from build123d import *

# Parameters (mm, degrees)
SKETCH_1_R                      = 4
EXTRUDE_1_DEPTH                 = 1
SKETCH_3_R                      = 2
EXTRUDE_3_DEPTH                 = 6.4
EXTRUDE_4_DEPTH                 = 2
CHAMFER_1_SIZE                  = 0.5
CHAMFER_2_SIZE                  = 1
CUT_EXTRUDE_1_REACH             = 10.542
CUT_EXTRUDE_1_DIRECTION_2_REACH = 10.542
EXTRUDE_START                   = 0.6
SKETCH_6_R                      = 4
EXTRUDE_5_DEPTH                 = 0.6
SKETCH_7_W                      = 8
SKETCH_7_H                      = 2
CUT_EXTRUDE_2_DEPTH             = 0.8


with BuildPart() as part:
    # 草图1 → 凸台-拉伸1 (new body)
    with BuildSketch(Plane(origin=(0, 0, 0), x_dir=(1, 0, 0), z_dir=(0, 1, 0))):
        with Locations(Location((0, 0, 0), (0, 0, 270))):
            Circle(SKETCH_1_R)
    extrude(amount=EXTRUDE_1_DEPTH)

    # 草图3 → 凸台-拉伸3 (add)
    with BuildSketch(Plane(origin=(0, 0, 0), x_dir=(-1, 0, 0), z_dir=(0, -1, 0))):
        with Locations(Location((0, 0, 0), (0, 0, 270))):
            Circle(SKETCH_3_R)
    extrude(amount=EXTRUDE_3_DEPTH)

    # 草图4 → 凸台-拉伸4 (add)
    with BuildSketch(Plane(origin=(0, -6.4, 0), x_dir=(-1, 0, 0), z_dir=(0, -1, 0))):
        with BuildLine():
            Line((2.598076211, -1.5), (-2.598076211, -1.5))
            ThreePointArc((-2.598076211, -1.5), (-3, 0), (-2.598076211, 1.5))
            Line((-2.598076211, 1.5), (2.598076211, 1.5))
            ThreePointArc((2.598076211, 1.5), (3, 0), (2.598076211, -1.5))
        make_face()
    extrude(amount=-EXTRUDE_4_DEPTH)

    # 倒角1
    chamfer_1_edges = [part.edges().sort_by_distance(p)[0] for p in [
        (3, -6.4, 0),
        (-3, -6.4, 0),
    ]]
    chamfer(chamfer_1_edges, length=CHAMFER_1_SIZE)

    # 倒角2
    chamfer_2_edges = [part.edges().sort_by_distance(p)[0] for p in [
        (3, -4.4, 0),
        (-3, -4.4, 0),
    ]]
    chamfer(chamfer_2_edges, length=CHAMFER_2_SIZE - 0.0001)  # a hair under: the kernel refuses the full size

    # 草图5 → 切除-拉伸1 (cut, up to next)
    with BuildSketch(Plane(origin=(0, 0, 0), x_dir=(0, 0, -1), z_dir=(1, 0, 0)), mode=Mode.PRIVATE) as cut_extrude_1_sk1:
        Polygon((2, -5.2), (1, -6.4), (2, -6.4), align=None)
    cut_extrude_1_tool1 = extrude(cut_extrude_1_sk1.sketch, amount=-CUT_EXTRUDE_1_REACH, mode=Mode.PRIVATE) & part.part
    # 草图5 → 切除-拉伸1 (cut, up to next)
    with BuildSketch(Plane(origin=(0, 0, 0), x_dir=(0, 0, -1), z_dir=(1, 0, 0)), mode=Mode.PRIVATE) as cut_extrude_1_sk2:
        Polygon((-2, -5.2), (-2, -6.4), (-1, -6.4), align=None)
    cut_extrude_1_tool2 = extrude(cut_extrude_1_sk2.sketch, amount=-CUT_EXTRUDE_1_REACH, mode=Mode.PRIVATE) & part.part
    add(cut_extrude_1_tool1.solids().sort_by_distance((0, -6, -1.666667))[0], mode=Mode.SUBTRACT)
    add(cut_extrude_1_tool2.solids().sort_by_distance((0, -6, 1.666667))[0], mode=Mode.SUBTRACT)

    # 草图5 → 切除-拉伸1 direction 2 (cut, up to next)
    with BuildSketch(Plane(origin=(0, 0, 0), x_dir=(0, 0, -1), z_dir=(1, 0, 0)), mode=Mode.PRIVATE) as cut_extrude_1_direction_2_sk1:
        Polygon((2, -5.2), (1, -6.4), (2, -6.4), align=None)
    cut_extrude_1_direction_2_tool1 = extrude(cut_extrude_1_direction_2_sk1.sketch, amount=CUT_EXTRUDE_1_DIRECTION_2_REACH, mode=Mode.PRIVATE) & part.part
    # 草图5 → 切除-拉伸1 direction 2 (cut, up to next)
    with BuildSketch(Plane(origin=(0, 0, 0), x_dir=(0, 0, -1), z_dir=(1, 0, 0)), mode=Mode.PRIVATE) as cut_extrude_1_direction_2_sk2:
        Polygon((-2, -5.2), (-2, -6.4), (-1, -6.4), align=None)
    cut_extrude_1_direction_2_tool2 = extrude(cut_extrude_1_direction_2_sk2.sketch, amount=CUT_EXTRUDE_1_DIRECTION_2_REACH, mode=Mode.PRIVATE) & part.part
    add(cut_extrude_1_direction_2_tool1.solids().sort_by_distance((0, -6, -1.666667))[0], mode=Mode.SUBTRACT)
    add(cut_extrude_1_direction_2_tool2.solids().sort_by_distance((0, -6, 1.666667))[0], mode=Mode.SUBTRACT)

    # 草图6 → 凸台-拉伸5 (add)
    with BuildSketch(Plane.XZ.offset(EXTRUDE_START)):
        with Locations(Location((0, 0, 0), (0, 0, 270))):
            Circle(SKETCH_6_R)
    extrude(amount=-EXTRUDE_5_DEPTH)

    # 草图7 → 切除-拉伸2 (cut)
    with BuildSketch(Plane(origin=(0, 1, 0), x_dir=(1, 0, 0), z_dir=(0, 1, 0))):
        Rectangle(SKETCH_7_W, SKETCH_7_H)
    extrude(amount=-CUT_EXTRUDE_2_DEPTH, mode=Mode.SUBTRACT)


solid = part.part
Part model, mm, in its own coordinate system. A direction names the side the tool comes from. Round coordinates to 2 decimals unless told otherwise and drop trailing zeros. Write each loop counter-clockwise with the first axis right and the second up, starting at its lowest first coordinate (ties: lowest second). Pieces come first, ordered by that corner, then holes. Notation, with made-up numbers: M 57,44.5 L 89,44.5 A19 ccw 89,56.5 Z; hole C -13.75,11 d8. An arc over 180 degrees is marked long. Return JSON: item names as keys, results as strings. Group by question number.
(1) Drill centre lines: probe 1 along Y at (x, z) = (0.5, 2.25); probe 2 along Y at (x, z) = (0.75, -0.5); probe 3 along Z at (x, y) = (0, -4). Where is each one in solid material? Low to high.
(2) Pin check, flat tips, straight feed: pin 1 Ø1 at (x, y) = (2, -5) entering from -Z; pin 2 Ø0.6 at (x, z) = (0.5, 0) entering from +Y; pin 3 Ø1.5 at (x, y) = (1.5, -4) entering from +Z. Stop position of each tip, or through.
(3) Saw through at C-C on y = -3.75. Write the cut outline in (x, z), then the cut area to 3 significant figures.
(4) Which spindle directions (+Z, -Z, +X, -X, +Y, -Y) get a long thin tool onto all of the face, cutting with end or side? Do faces 1 (the face through (-2.4, -4.8, 0)), 2 (the face through (-1, -0.6, 2)), 3 (the face through (-1.8, -5.3, 1.5)), 4 (the face through (1.8, -5.3, -1.5)), 5 (the face through (0, 0.2, 0)). Say none if no direction does.
(5) Saw through at A-A on x = 0. Write the cut outline in (y, z).
(6) Saw through at D-D on x = 1. Write the cut outline in (y, z), then the cut area to 3 significant figures.
(7) Saw through at B-B on z = 1.75. Write the cut outline in (x, y), then the cut area to 3 significant figures.
(8) Two-plate mould, pull along Y, no slides. Class faces 6 (the face through (2, -3, 0)), 7 (the face through (-1.8, -5.3, -1.5)), 8 (the face through (0, 1, 2)): +Y half, -Y half, draft (parallel to the pull), parting line (faces both ways), or undercut.
Returned:
{
 "1": {"probe 1": "-0.6 to 1", "probe 2": "-6.4 to 0.2", "probe 3": "-2 to 2"},
 "2": {"pin 1": "z = -1.5", "pin 2": "y = 0.2", "pin 3": "z = 1.85"},
 "3": {"outline": "C 0,0 d4", "area": "12.6 mm²"},
 "4": {"face 1": "-X", "face 2": "none", "face 3": "+Z, -X, -Y", "face 4": "-Z, +X, -Y", "face 5": "+X, -X, +Y"},
 "5": {"outline": "M -6.4,-1 L -5.2,-2 L -0.6,-2 L -0.6,-4 L 1,-4 L 1,-1 L 0.2,-1 L 0.2,1 L 1,1 L 1,4 L -0.6,4 L -0.6,2 L -5.2,2 L -6.4,1 Z"},
 "6": {"outline": "M -6.4,-1 L -5.52,-1.73 L -0.6,-1.73 L -0.6,-3.87 L 1,-3.87 L 1,-1 L 0.2,-1 L 0.2,1 L 1,1 L 1,3.87 L -0.6,3.87 L -0.6,1.73 L -5.52,1.73 L -6.4,1 Z", "area": "30.2 mm²"},
 "7": {"outline": "M -3.6,-0.6 L -0.97,-0.6 L -0.97,-5.5 L 0.97,-5.5 L 0.97,-0.6 L 3.6,-0.6 L 3.6,1 L -3.6,1 Z", "area": "21.0 mm²"},
 "8": {"face 6": "undercut", "face 7": "draft", "face 8": "+Y half"}
}
